Autodesk Inventor part; units mm, degrees
ref_plane "YZ Plane" through (0, 0, 0) normal (1, 0, 0) x (0, 1, 0)
ref_plane "XZ Plane" through (0, 0, 0) normal (0, 1, 0) x (-1, 0, 0)
ref_plane "XY Plane" through (0, 0, 0) normal (0, 0, 1) x (1, 0, 0)
sketch "Sketch1" plane through (0, 0, 0) normal (0, 0, 1) x (1, 0, 0)
  line L0 (-12.1708, 16.0073) -> (13.2292, 16.0073)
  line L1 (13.2292, 16.0073) -> (13.2292, -34.7927)
  line L2 (13.2292, -34.7927) -> (-12.1708, -34.7927)
  line L3 (-12.1708, -34.7927) -> (-12.1708, 16.0073)
  line L4 (11.9592, 14.7373) -> (-10.9008, 14.7373)
  line L5 (-10.9008, 14.7373) -> (-10.9008, -33.5227)
  line L6 (-10.9008, -33.5227) -> (11.9592, -33.5227)
  line L7 (11.9592, -33.5227) -> (11.9592, 14.7373)
  point P0 (0, 0)
  dimension "d0" = 25.4
  dimension "d1" = 50.8
  dimension "d2" = 1.27
extrude "Extrusion1" add sketch "Sketch1" along normal blind 177.8
sketch "Sketch2" plane through (-12.1708, 16.0073, 0) normal (0, 1, 0) x (1, 0, 0)
  circle A0 centre (12.7, -12.7) radius 1.7272
  line L0 (25.4, 0) -> (0, 0)
  line L1 (0, 0) -> (0, -177.8)
  point P0 (12.1708, 0)
  dimension "d5" = 3.4544
  dimension "d6" = 12.7
  dimension "d7" = 12.7
extrude "Extrusion2" cut sketch "Sketch2" against normal through all
pattern_linear "Rectangular Pattern1" count 18 spacing 25.4 along (0, 0, 1) of "Extrusion2"
sketch "Sketch3" plane through (13.2292, -34.7927, 0) normal (1, 0, 0) x (0, 0, -1)
  circle A0 centre (-38.1, 25.4) radius 14.2875
  line L0 (0, 0) -> (-177.8, 0)
  line L1 (0, 0) -> (0, 50.8)
  circle A1 centre (-38.1, 25.4) radius 24.7523
  line L2 (-20.5975, 42.9025) -> (-55.6025, 42.9025)
  line L3 (-55.6025, 42.9025) -> (-55.6025, 7.8975)
  line L4 (-55.6025, 7.8975) -> (-20.5975, 7.8975)
  line L5 (-20.5975, 7.8975) -> (-20.5975, 42.9025)
  circle A2 centre (-20.5975, 42.9025) radius 2.159
  circle A3 centre (-20.5975, 7.8975) radius 2.159
  circle A4 centre (-55.6025, 7.8975) radius 2.159
  circle A5 centre (-55.6025, 42.9025) radius 2.159
  point P0 (0, 34.7927)
  point P1 (0, 25.4)
  dimension "d15" = 28.575
  dimension "d16" = 25.4
  dimension "d17" = 38.1
  dimension "d20" = 49.5046
  dimension "d22" = 4.318
  dimension "d23" = 4.318
  dimension "d24" = 4.318
  dimension "d25" = 4.318
extrude "Extrusion3" cut sketch "Sketch3" against normal blind 25.4 contours A0 | A2 L5 A1 | A1 A2 | A3 A1 | A1 L5 A3 | L2 A2 A1 | L5 A2 L2 | A1 A3 L4 | L4 A3 L5 | A5 L2 A1 | A1 A5 | A5 L3 L2 | A4 A1 | A1 L4 A4 | L4 L3 A4 | L3 A5 A1 | A1 A4 L3
equation "\"d3\" = d13"
equation "\"d23\" = d22"
equation "\"d24\" = d22"
equation "\"d25\" = d22"
equation "\"d10\" = d14"
equation "\"d13\" = 177.8"
equation "\"d14\" = d13"
properties part number "VersaFrame (Jumper Bar)"
The model under review builds one solid part; all positions refer to its coordinate system, in mm. A direction names the side the tool comes from. Give positions to 0.01 mm unless a question says otherwise; leave off trailing zeros. Write each loop counter-clockwise with the first axis right and the second up, starting at its lowest first coordinate (ties: lowest second). Pieces come first, ordered by that corner, then holes. Notation, with made-up numbers: M 49.5,-15.75 L 76.5,-15.75 A28 ccw 76.5,9.25 Z; hole C -1.75,-26.75 d7. An arc over 180 degrees is marked long. Write each question's results on one line, items separated by ' | '. Start each with the question number.
1. We need section A-A (z = 38.1). Write out the cut boundary in (x, y), and give its area (3 significant figures).
2. For probe 1 along Y at (x, z) = (6.5, 169.5); probe 2 along X at (y, z) = (-25, 44.5); probe 3 along X at (y, z) = (15.4, 12.7), list the stretches that pass through material, from the lowest coordinate up. Write a range as [from, to].
3. For faces 1 (the flat face through (-12.171, -10, 88)), 2 (the flat face through (3, -33.523, 88)), list the 3-axis set-ups (+Z, -Z, +X, -X, +Y, -Y) from which the entire face can be reached by the end or side of a thin tool; tool diameter is ignored.
4. We need section D-D (z = 161). Write out the cut boundary in (x, y), and give its area (3 significant figures).
5. Insertion check: pin 1 Ø3.5 at (y, z) = (-26.9, 20.6) entering from -X. The pin has a flat end and moves straight along its axis. Give the tip position at first contact, or say it passes through.
6. Mouldability with a two-part tool opening along Y and no side actions: class faces 3 (the flat face through (-12, -9, 0)), 4 (the cylindrical face through (-11.527, 8.758, 53.543)), 5 (the flat face through (4, -34.793, 88)) as released by +Y, released by -Y, zero draft, split by the parting line, or undercut.
7. We need section B-B (x = -8.25). Write out the cut boundary in (y, z), and give its area (3 significant figures).
8. We need section C-C (y = 0). Write out the cut boundary in (x, z), and give its area (3 significant figures).
Results found:
1) outline: M -12.17,-34.79 L -1.2,-34.79 L -1.2,-33.52 L -10.9,-33.52 L -10.9,-23.68 L -12.17,-23.68 Z; M -12.17,4.89 L -10.9,4.89 L -10.9,14.74 L -1.2,14.74 L -1.2,16.01 L -12.17,16.01 Z; M 2.26,-34.79 L 13.23,-34.79 L 13.23,-23.68 L 11.96,-23.68 L 11.96,-33.52 L 2.26,-33.52 Z; M 2.26,14.74 L 11.96,14.74 L 11.96,4.89 L 13.23,4.89 L 13.23,16.01 L 2.26,16.01 Z | area: 106 mm^2
2) probe 1: y = [-34.79, -33.52], [14.74, 16.01] | probe 2: x = [-12.17, -10.9], [11.96, 13.23] | probe 3: x = [-12.17, -1.2], [2.26, 13.23]
3) face 1: +Z, -Z, -X, +Y, -Y | face 2: +Z, -Z
4) outline: M -12.17,-34.79 L 13.23,-34.79 L 13.23,16.01 L -12.17,16.01 Z; hole M -10.9,-33.52 L 11.96,-33.52 L 11.96,14.74 L -10.9,14.74 Z | area: 187 mm^2
5) pin 1: passes through
6) face 3: zero draft | face 4: undercut | face 5: released by -Y
7) outline: M -34.79,0 L -33.52,0 L -33.52,177.8 L -34.79,177.8 Z; M 14.74,0 L 16.01,0 L 16.01,177.8 L 14.74,177.8 Z | area: 452 mm^2
8) outline: M -12.17,0 L -10.9,0 L -10.9,27.33 L -12.17,27.33 Z; M -12.17,48.87 L -10.9,48.87 L -10.9,177.8 L -12.17,177.8 Z; M 11.96,0 L 13.23,0 L 13.23,27.33 L 11.96,27.33 Z; M 11.96,48.87 L 13.23,48.87 L 13.23,177.8 L 11.96,177.8 Z | area: 397 mm^2
